Autodesk Inventor part; units mm, degrees
ref_plane "YZ Plane" through (0, 0, 0) normal (1, 0, 0) x (0, 1, 0)
ref_plane "XZ Plane" through (0, 0, 0) normal (0, 1, 0) x (-1, 0, 0)
ref_plane "XY Plane" through (0, 0, 0) normal (0, 0, 1) x (1, 0, 0)
sketch "Sketch1" plane through (0, 0, 0) normal (0, 1, 0) x (-1, 0, 0)
  line L0 (0, 0) -> (444.5, 0)
  line L1 (444.5, 0) -> (444.5, -444.5)
  line L2 (444.5, -444.5) -> (0, -444.5)
  line L3 (0, -444.5) -> (0, 0)
  dimension "d0" = 444.5
  dimension "d1" = 444.5
extrude "Extrusion1" add sketch "Sketch1" along normal blind 6.35
sketch "Sketch2" plane through (0, 6.35, 0) normal (0, 1, 0) x (1, 0, 0)
  line L0 (-444.5, 0) -> (0, 0)
  line L1 (-444.5, 444.5) -> (-444.5, 0)
  line L2 (-419.1, 304.8) -> (-419.1, 139.7) construction
  line L3 (-431.8, 292.1) -> (-431.8, 152.4)
  line L4 (-406.4, 152.4) -> (-406.4, 292.1)
  arc A0 (-406.4, 292.1) -> (-431.8, 292.1) centre (-419.1, 292.1) ccw
  arc A1 (-431.8, 152.4) -> (-406.4, 152.4) centre (-419.1, 152.4) ccw
  line L5 (0, 444.5) -> (-444.5, 444.5)
  point P0 (-419.1, 222.25)
  dimension "d8" = 444.5
  dimension "d12" = 25.4
  dimension "d13" = 12.7
  dimension "d14" = 165.1
  dimension "d15" = 139.7
extrude "Extrusion3" cut sketch "Sketch2" against normal through all
equation "\"d15\" = -0.5 * d14 + 0.5 * d8"
properties part number "Top Plate" material "Nylon 6/6"
Design review of the part built by this model. Coordinates are the model's own, in mm. A direction names the side the tool comes from. Round coordinates to 2 decimals unless told otherwise and drop trailing zeros. Write each loop counter-clockwise with the first axis right and the second up, starting at its lowest first coordinate (ties: lowest second). Pieces come first, ordered by that corner, then holes. Notation, with made-up numbers: M -7,52 L 52,52 A27 ccw 52,68 Z; hole C -35.5,79.5 d9. An arc over 180 degrees is marked long. One line per item, written item: value. Start each with the question number.
1. Take a section at A-A on z = -163. State the section outline as (x, y) points.
2. For faces 3 (the face through (-419.379, 3.219, -139.703)), 4 (the face through (-219, 0, -219)), list the 3-axis set-ups (+Z, -Z, +X, -X, +Y, -Y) from which the entire face can be reached by the end or side of a thin tool; tool diameter is ignored.
3. Draft analysis for pull direction X (two halves, no side actions). For faces 1 (the face through (-219, 6.35, -219)), 2 (the face through (-418.821, 3.219, -304.797)), state which applies: pulls with the +X half, pulls with the -X half, needs draft (parallel to the pull), parting line crosses it, or undercut.
4. Take a section at C-C on y = 3.75. State the section outline as (x, z) points.
5. Clearance check with a flat-ended pin moving along its axis: P1, Ø3, axis at y = 4, z = -308.5, coming from the +X side. State where the tip first meets the part, or that it passes through.
6. Take a section at B-B on x = -419.1. State the section outline as (y, z) points.
7. To check wall thickness, follow probe 1 along X at (y, z) = (4.25, -280); probe 2 along Z at (x, y) = (-422.5, 5.5). State the ranges of each line that lie inside material, in increasing order. Write a range as from..to.
Computed:
1. outline: M -444.5,0 L -431.8,0 L -431.8,6.35 L -444.5,6.35 Z; M -406.4,0 L 0,0 L 0,6.35 L -406.4,6.35 Z
2. face 3: +Y, -Y
2. face 4: +Z, -Z, +X, -X, -Y
3. face 1: needs draft
3. face 2: undercut
4. outline: M -444.5,-444.5 L 0,-444.5 L 0,0 L -444.5,0 Z; hole M -431.8,-292.1 A12.7 ccw -406.4,-292.1 L -406.4,-152.4 A12.7 ccw -431.8,-152.4 Z
5. P1: stops at x = 0
6. outline: M 0,-444.5 L 6.35,-444.5 L 6.35,-304.8 L 0,-304.8 Z; M 0,-139.7 L 6.35,-139.7 L 6.35,0 L 0,0 Z
7. probe 1: x = -444.5..-431.8, -406.4..0
7. probe 2: z = -444.5..-304.34, -140.16..0
